Input: part model. Units: mm. Frame: model coordinates. A direction names the side the tool comes from. Round coordinates to 2 decimals unless told otherwise and drop trailing zeros. Write each loop counter-clockwise with the first axis right and the second up, starting at its lowest first coordinate (ties: lowest second). Pieces come first, ordered by that corner, then holes. Notation, with made-up numbers: (75, -32) - (116, -32) arc R16 cw to (116, -21) - close; hole circle Ø11 at (-38.75, -19). An arc over 180 degrees is marked (long way). Use one line per item in the form item = value.
Autodesk Fusion 360 part; units mm, degrees
sketch "Sketch1" plane through (0, 0, 0) normal (0, 1, 0) x (1, 0, 0)
  line L0 (22, 19) -> (-16, 19)
  line L1 (-16, 19) -> (-16, 0)
  line L2 (-16, 0) -> (0, 0)
  line L3 (0, 0) -> (0, -11.1807)
  arc A0 (0, -11.1807) -> (22, -36) centre (25, -11.1807) ccw
  line L4 (22, -36) -> (22, 19)
  dimension "d1" = 55
  dimension "d2" = 38
  dimension "d3" = 25
  dimension "d4" = 16
  dimension "d5" = 19
extrude "Extrude1" add sketch "Sketch1" along normal blind 34 and the other way blind 34
sketch "Sketch2" plane through (-16, 0, 0) normal (-1, 0, 0) x (0, -1, 0)
  line L0 (34, 0) -> (-34, 0)
  line L1 (-34, 0) -> (-34, -19)
  line L2 (-34, -19) -> (34, -19)
  line L3 (34, -19) -> (34, 0)
  line L4 (-12, -19) -> (12, -19)
  line L5 (12, -19) -> (12, -31)
  line L6 (12, -31) -> (-12, -31)
  line L7 (-12, -31) -> (-12, -19)
  dimension "d10" = 12
  dimension "d11" = 24
  dimension "d12" = 22
extrude "Extrude2" add sketch "Sketch2" against normal blind 95 contours L2 L4 L5 L6 L7
chamfer "Chamfer1" distance 12 distance2 6 1 edges at (79, 0, -19) measured on face at (79, 4, -23)
sketch "Sketch3" plane through (-16, 0, 0) normal (-1, 0, 0) x (0, -1, 0)
  line L0 (34, 0) -> (-34, 0)
  line L1 (-34, 0) -> (-34, -19)
  line L2 (-34, -19) -> (-12, -19)
  line L3 (-12, -19) -> (-12, -31)
  line L4 (-12, -31) -> (12, -31)
  line L5 (12, -31) -> (12, -19)
  line L6 (12, -19) -> (34, -19)
  line L7 (34, -19) -> (34, 0)
  arc A0 (16, 0) -> (-16, 0) centre (0, 0) ccw
  dimension "d17" = 32
extrude "Extrude3" add sketch "Sketch3" along normal up to surface contours L0 A0 end surface at (1.4183, 11.3333, 19.4813)
sketch "Sketch4" plane through (-16, 0, 0) normal (-1, 0, 0) x (0, -1, 0)
  line L0 (34, 0) -> (16, 0)
  arc A0 (16, 0) -> (-16, 0) centre (0, 0) ccw
  line L1 (-16, 0) -> (-34, 0)
  line L2 (-34, 0) -> (-34, -19)
  line L3 (-34, -19) -> (-12, -19)
  line L4 (-12, -19) -> (-12, -31)
  line L5 (-12, -31) -> (12, -31)
  line L6 (12, -31) -> (12, -19)
  line L7 (12, -19) -> (34, -19)
  line L8 (34, -19) -> (34, 0)
  circle A1 centre (0, 0) radius 6
  dimension "d21" = 12
extrude "Extrude4" cut sketch "Sketch4" against normal blind 16 contours A1
(1) Cut plane C-C on z = 13. Output: boundary loops of the cut face in (x, y), then the cut area to 3 significant figures.
Derived:
outline = (-16, -9.33) - (0.07, -9.33) - (0.07, -34) - (22, -34) - (22, 34) - (0.07, 34) - (0.07, 9.33) - (-16, 9.33) - close
area = 1,790 mm^2
(2) Cut plane B-B on x = 62. Output: boundary loops of the cut face in (y, z), then the cut area to 3 significant figures.
Derived:
outline = (-12, -31) - (12, -31) - (12, -19) - (-12, -19) - close
area = 288 mm^2
(3) Access query for faces 1 (the face through (-8, 0, 16)), 2 (the face through (3, 23, -19)), 3 (the face through (-8, -25, 0)), 4 (the face through (22, 0, 9)). Directions: +Z, -Z, +X, -X, +Y, -Y. A direction counts if a zero-diameter tool reaches every point of the face in a straight line with its end or side. Return the directions, or none.
Derived:
face_1 = +Z, -X
face_2 = -Z, +X, -X, +Y
face_3 = +Z, -X, -Y
face_4 = +Z, +X, +Y, -Y
(4) Draft query along Z for faces 5 (the face through (31, 0, -31)), 6 (the face through (76, 0, -25)), 7 (the face through (0, 0, 0)). Return one class per face: released by +Z, released by -Z, zero draft, split by the parting line, or undercut.
Derived:
face_5 = released by -Z
face_6 = released by +Z
face_7 = undercut
(5) Cut plane A-A on y = 26. Output: boundary loops of the cut face in (x, z), then the cut area to 3 significant figures.
Derived:
outline = (-16, -19) - (22, -19) - (22, 36) arc R25 ccw to (0, 11.18) - (0, 0) - (-16, 0) - close
area = 1,380 mm^2
(6) First-contact query: pin 1 Ø12 at (x, y) = (39.5, 2) entering from +Z; pin 2 Ø3.5 at (x, z) = (44.5, -26.5) entering from -Y; pin 3 Ø6 at (y, z) = (25.5, -5) entering from +X. Flat tips, straight axial feed; report the tip coordinate or a pass-through.
Derived:
pin_1 = -19
pin_2 = -12
pin_3 = 22
(7) Material intervals for L1, parallel to Z at x = -3, y = 0; L2, parallel to Z at x = 67, y = 1.5; L3, parallel to X at y = 15, z = -12, sorted ascending.
Derived:
L1 = -31 to -6, 6 to 16
L2 = -31 to -19
L3 = -16 to 22
